Build history of the part. All positions in model axes, mm. A direction names the side the tool comes from. Give positions to 0.01 mm unless a question says otherwise; leave off trailing zeros. Order: outer loops, then holes, each group sorted by start corner. A loop starts at its lowest first (then second) coordinate and runs counter-clockwise, first axis right, second up. Notation, with made-up numbers: M 84,5 L 113,5 A28 cw 113,37 Z; hole C -5,79.25 d11. An arc over 180 degrees is marked long. Use CSV: the item, a comma, the result in double quotes. Start each with the question number.
Item 1: Band-saw the part on A-A on x = 90. Write the cut outline in (y, z).
Item 2: Band-saw the part on C-C on z = -15.5. Write the cut outline in (x, y), plus the area to 3 significant figures.
Item 3: Wall check: line 1 along X through (y, z) = (-33.5, 27.5); line 2 along X through (y, z) = (33, -29.5); line 3 along X through (y, z) = (23, 25). Give the ranges that are in metal, low to high.
Item 4: Band-saw the part on B-B on y = 135. Write the cut outline in (x, z).
Item 5: Two-plate mould, pull along Z, no slides. Class faces 6 (the flat face through (22, 50.8, 27)), 7 (the flat face through (-6.35, 77, 19)), 8 (the flat face through (51, -9, 50.8)): pulls with the +Z half, pulls with the -Z half, needs draft (parallel to the pull), parting line crosses it, or undercut.
Item 6: Pin check, flat tips, straight feed: P1, Ø10, axis at y = -69.5, z = 26.5, coming from the -X side; P2, Ø15.5, axis at x = 19.5, z = 31, coming from the +Y side; P3, Ø20.5, axis at y = -17.5, z = 30, coming from the -X side; P4, Ø4, axis at y = 68.5, z = 23.5, coming from the -X side. Stop position of each tip, or through.
Item 7: Band-saw the part on D-D on x = 58.5. Write the cut outline in (y, z).
Item 8: Which spindle directions (+Z, -Z, +X, -X, +Y, -Y) get a long thin tool onto all of the face, cutting with end or side? Do faces 1 (the flat face through (101.6, -13, 25)), 2 (the cylindrical face through (-3.774, 94.267, 31.41)), 3 (the cylindrical face through (-63.411, 65.155, 26.311)), 4 (the flat face through (0, -13, 25)), 5 (the flat face through (50, -13, 0)). Say none if no direction does.
from build123d import *

# Parameters (mm, degrees)
F0_W      = 101.6
F0_H      = 50.8
F1_DEPTH  = 25.4
F3_DEPTH  = 76.2
F4_R      = 7.4724872864
F5_DEPTH  = 50.8
F6_R      = 28.3895179235
F6_R_2    = 7.4724872864
F7_DEPTH  = 6.35
F8_SIZE   = 12.69999
F9_R      = 23.7493356576
F10_DEPTH = 6.35
F11_SIZE  = 7.62
F12_R     = 6.7723102527
F13_DEPTH = 50.8
F14_R     = 82.1200007596
F14_R_2   = 6.7723102527
F15_DEPTH = 12.7


# Not quite as in the source:
# - a fillet or chamfer is up to 0.001 mm smaller than in the source, because OpenCascade refuses the exact size


with BuildPart() as f1:
    # F0 (on Front) → F1 (new body)
    with BuildSketch(Plane.XZ):
        with Locations((50.8, 25.4)):
            Rectangle(F0_W, F0_H)
    extrude(amount=F1_DEPTH)

    # F2 (on face) → F3 (join)
    with BuildSketch(Plane.XZ.offset(25.4)):
        with BuildLine():
            ThreePointArc((73.4443714217, 50.8), (58.5934004133, 10.4401432835), (98.1016742507, 27.4273641407))
            ThreePointArc((98.1016742507, 27.4273641407), (91.6827931143, 43.5295359845), (75.9467730924, 50.8))
            Line((75.9467730924, 50.8), (73.4443714217, 50.8))
        make_face()
    extrude(amount=F3_DEPTH)

    # F4 (on face) → F5 (join)
    with BuildSketch(Plane(origin=(0, 0, 0), x_dir=(-1, 0, 0), z_dir=(0, 1, 0))):
        with Locations((-21.7883531004, 26.4536123723)):
            Circle(F4_R)
    extrude(amount=F5_DEPTH)

    # F6 (on face) → F7 (join, symmetric)
    with BuildSketch(Plane(origin=(0, 50.8, 0), x_dir=(-1, 0, 0), z_dir=(0, 1, 0))):
        with Locations((-21.7883531004, 26.4536123723)):
            Circle(F6_R)
        with Locations((-21.7883531004, 26.4536123723)):
            Circle(F6_R_2, mode=Mode.SUBTRACT)
    extrude(amount=F7_DEPTH, both=True)

    # F8 (size 12.7 in the source; OpenCascade refuses exactly that, so slightly less here)
    f8_edges = [f1.edges().sort_by_distance(p)[0] for p in [
        (50.177871, 57.15, 26.453612),
    ]]
    chamfer(f8_edges, length=F8_SIZE)

    # F9 (on Right) → F10 (join, symmetric)
    with BuildSketch(Plane.YZ):
        with Locations((71.6144831948, 24.2767716783)):
            Circle(F9_R)
    extrude(amount=F10_DEPTH, both=True)

    # F11
    f11_edges = [f1.edges().sort_by_distance(p)[0] for p in [
        (6.35, 79.39333, 46.716034),
        (6.35, 78.162989, 1.448105),
    ]]
    chamfer(f11_edges, length=F11_SIZE)

    # F12 (on face) → F13 (join)
    with BuildSketch(Plane(origin=(-6.35, 0, 0), x_dir=(0, -1, 0), z_dir=(-1, 0, 0))):
        with Locations((-71.6144831948, 24.2767716783)):
            Circle(F12_R)
    extrude(amount=F13_DEPTH)

    # F14 (on face) → F15 (join, symmetric)
    with BuildSketch(Plane(origin=(-57.15, 0, 0), x_dir=(0, -1, 0), z_dir=(-1, 0, 0))):
        with Locations((-71.6144831948, 24.2767716783)):
            Circle(F14_R)
        with Locations((-71.6144831948, 24.2767716783)):
            Circle(F14_R_2, mode=Mode.SUBTRACT)
    extrude(amount=F15_DEPTH, both=True)


solid = f1.part
Model answer:
1,outline,"M -101.6,9.72 L -25.4,9.72 L -25.4,0 L 0,0 L 0,50.8 L -25.4,50.8 L -25.4,45.14 L -101.6,45.14 Z"
2,outline,"M -69.85,-0.23 L -44.45,-0.23 L -44.45,143.46 L -69.85,143.46 Z"
2,area,"3,650 mm^2"
3,line 1,"x = 51.29 to 98.1"
3,line 2,"x = -69.85 to -44.45"
3,line 3,"x = -69.85 to -44.45, 14.46 to 29.12"
4,outline,"M -69.85,-27.93 L -44.45,-27.93 L -44.45,76.49 L -69.85,76.49 Z"
5,face 6,"undercut"
5,face 7,"needs draft"
5,face 8,"pulls with the +Z half"
6,P1,"stops at x = 51.29"
6,P2,"stops at y = 57.15"
6,P3,"stops at x = -69.85"
6,P4,"stops at x = -57.15"
7,outline,"M -101.6,10.53 L -25.4,10.53 L -25.4,0 L 0,0 L 0,50.8 L -25.4,50.8 L -25.4,44.33 L -101.6,44.33 Z"
8,face 1,"+Z, -Z, +X, +Y, -Y"
8,face 2,"none"
8,face 3,"-X"
8,face 4,"+Z, -Z, -Y"
8,face 5,"-Z, +X, -Y"
